Could you check a few things on this model? Use its own coordinates, in mm. A direction names the side the tool comes from. Round coordinates to 2 decimals unless told otherwise and drop trailing zeros. Write each loop counter-clockwise with the first axis right and the second up, starting at its lowest first coordinate (ties: lowest second). Pieces come first, ordered by that corner, then holes. Notation, with made-up numbers: (55, -14.5) - (99, -14.5) arc R12 ccw to (99, -1.5) - close; hole circle Ø5 at (58.5, 50). An arc over 180 degrees is marked (long way). Write each question's results on one line, items separated by ' | '. Start each with the question number.
(1) For P1, Ø3, axis at x = 144.5, z = 5, coming from the -Y side; P2, Ø3, axis at x = -36.5, z = 3.5, coming from the -Y side; P3, Ø1, axis at y = -22, z = 8.5, coming from the +X side; P4, Ø17, axis at x = 188.14, y = 86.98, coming from the -Z side, each with a flat end and sliding along its axis, tell me the tip position at first contact or that it passes through.
(2) Imagine slicing it at C-C on x = -39. Write out the boundary of the cut face in (y, z).
(3) Please list where these lines run through material, in increasing order: line 1 (X direction, y = 200.5, z = 1.5); line 2 (Y direction, x = 198, z = 6.5); line 3 (X direction, y = 167, z = 2.5). Write a range as [from, to].
(4) Thinking about a two-plate mould opening in Y: for faces 1 (the cylindrical face through (223.75, 216.01, 4.93)), 2 (the cylindrical face through (194.343, 88.932, 4.93)), 3 (the flat face through (-142, -153.506, 5)), which applies, +Y half, -Y half, draft (parallel to the pull), parting line (faces both ways), or undercut?
(5) On a 3-axis mill with a long thin cutter (end or side, diameter ignored), from which of +Z, -Z, +X, -X, +Y, -Y can I reach the whole of each face in a straight line? I mean faces 4 (the flat face through (148.305, 162, 5)), 5 (the cylindrical face through (197.884, 162.629, 4.93)), 6 (the flat face through (-135.04, -137.9, 4.93)). Say none if no direction works.
(6) Imagine slicing it at A-A on z = 5. Write out the boundary of the cut face in (x, y), then the cut area to 3 significant figures.
(7) Imagine slicing it at B-B on y = 146.5. Write out the boundary of the cut face in (x, z), then the cut area to 3 significant figures.
```python
from build123d import *

# Parameters (mm, degrees)
F0_R     = 6.5
F0_R_2   = 20
F1_DEPTH = 10


with BuildPart() as f1:
    # F0 (on Top) → F1 (new body)
    with BuildSketch(Plane.XY):
        with BuildLine():
            Line((140.366762, 103.505751), (-158.918484, -56.188821))
            ThreePointArc((-158.918484, -56.188821), (-164.720206, -61.706555), (-166.857052, -69.422724))
            Line((-166.857052, -69.422724), (-166.857052, -138.506076))
            ThreePointArc((-166.857052, -138.506076), (-165.180916, -145.396261), (-160.527098, -150.746595))
            ThreePointArc((-160.527098, -150.746595), (-156.40635, -152.799567), (-151.857052, -153.506076))
            Line((-151.857052, -153.506076), (-142.060088, -153.506076))
            Line((-142.060088, -153.506076), (-131.857052, -153.506076))
            Line((-131.857052, -153.506076), (-138.314184, -121.846012))
            ThreePointArc((-138.314184, -121.846012), (-135.860571, -113.930547), (-129.578516, -108.525866))
            Line((-129.578516, -108.525866), (219.285821, 51.720148))
            ThreePointArc((219.285821, 51.720148), (225.630142, 57.220563), (228.024481, 65.268676))
            Line((228.024481, 65.268676), (228.024481, 205.523393))
            ThreePointArc((228.024481, 205.523393), (223.631082, 216.129995), (213.024481, 220.523393))
            Line((213.024481, 220.523393), (163.305104, 220.523393))
            ThreePointArc((163.305104, 220.523393), (152.698503, 216.129995), (148.305104, 205.523393))
            Line((148.305104, 205.523393), (148.305104, 116.657392))
            ThreePointArc((148.305104, 116.657392), (146.147278, 108.988242), (140.366762, 103.505751))
        make_face()
        with Locations((188.142948, 86.979855)):
            Circle(F0_R, mode=Mode.SUBTRACT)
        with Locations((188.655132, 180.372253)):
            Circle(F0_R_2, mode=Mode.SUBTRACT)
    extrude(amount=F1_DEPTH)


solid = f1.part
```
Response:
1) P1: y = 16.68 | P2: y = -66.46 | P3: x = 59.88 | P4: z = 0
2) outline: (-66.92, 0) - (7.8, 0) - (7.8, 10) - (-66.92, 10) - close
3) line 1: [148.31, 228.02] | line 2: [41.94, 162.69], [198.05, 220.52] | line 3: [148.31, 173.78], [203.53, 228.02]
4) face 1: +Y half | face 2: undercut | face 3: -Y half
5) face 4: +Z, -Z, -X, +Y | face 5: +Z, -Z | face 6: +Z, -Z, +X
6) outline: (-166.86, -138.51) arc R15 ccw to (-160.53, -150.75) arc R15 ccw to (-151.86, -153.51) - (-131.86, -153.51) - (-138.31, -121.85) arc R15 cw to (-129.58, -108.53) - (219.29, 51.72) arc R15 ccw to (228.02, 65.27) - (228.02, 205.52) arc R15 ccw to (213.02, 220.52) - (163.31, 220.52) arc R15 ccw to (148.31, 205.52) - (148.31, 116.66) arc R15 cw to (140.37, 103.51) - (-158.92, -56.19) arc R15 ccw to (-166.86, -69.42) - close; hole circle Ø40 at (188.66, 180.37); hole circle Ø13 at (188.14, 86.98) | area: 38,400 mm²
7) outline: (148.31, 0) - (228.02, 0) - (228.02, 10) - (148.31, 10) - close | area: 797 mm²
